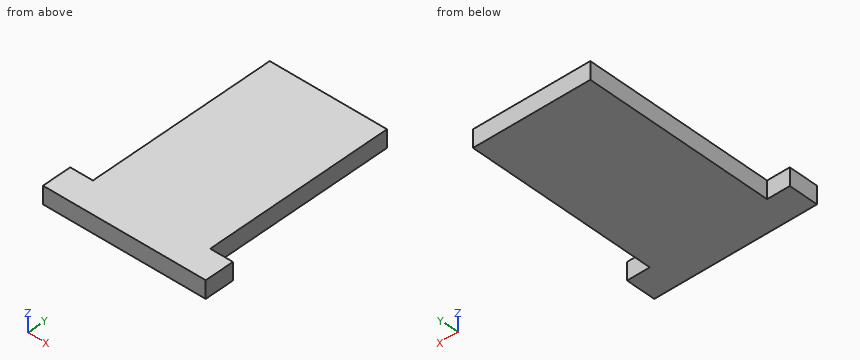
```python
from build123d import *

# Parameters (mm, degrees)
SKETCH1_W           = 8
SKETCH1_H           = 13
BOSS_EXTRUDE1_DEPTH = 0.6
SKETCH2_W           = 11.1
SKETCH2_H           = 2
BOSS_EXTRUDE2_DEPTH = 1.2


with BuildPart() as part:
    # Sketch1 → Boss-Extrude1 (new, symmetric)
    with BuildSketch(Plane.XY):
        Rectangle(SKETCH1_W, SKETCH1_H)
    extrude(amount=BOSS_EXTRUDE1_DEPTH, both=True)

    # Sketch2 → Boss-Extrude2 (add)
    with BuildSketch(Plane.XY.offset(0.6)):
        with Locations((0, -7.5)):
            Rectangle(SKETCH2_W, SKETCH2_H)
    extrude(amount=-BOSS_EXTRUDE2_DEPTH)


solid = part.part
```
The listing builds one solid part. Answer for the finished solid, in the listing's coordinates (mm). Give positions to 0.01 mm unless a question says otherwise; leave off trailing zeros. Loops run counter-clockwise (first coordinate to the right, second up) from the corner with the lowest first, then second, coordinate; pieces in that order, holes last. Notation, with made-up numbers: (-1.75, 84.5) - (17.25, 84.5) arc R15 ccw to (17.25, 102.5) - close; hole circle Ø1 at (2.25, -37). An arc over 180 degrees is marked (long way). Answer as CSV lines item,"result". Start each with the question number.
Item 1: A cutting plane is placed at A-A on z = 0.35. Determine the outline of the cut face in (x, y), then the cut area to 3 significant figures.
Item 2: Each of these flat-tipped pins is pushed along its axis until it touches: pin 1 (0.6 mm diameter, centred on y = -3, z = 0, fed in from +X); pin 2 (0.6 mm diameter, centred on x = 5, z = 0, fed in from +Y); pin 3 (2 mm diameter, centred on x = -4.5, y = -0.5, fed in from +Z). Where does it stop, or does it pass through?
Item 3: Find the intervals of material crossed by line 1 (X direction, y = -1.75, z = -0.15); line 2 (Y direction, x = 5, z = 0), in increasing order. Write a range as from..to.
Item 4: A cutting plane is placed at C-C on y = -2. Determine the outline of the cut face in (x, z), then the cut area to 3 significant figures.
Item 5: A cutting plane is placed at B-B on x = 4.5. Determine the outline of the cut face in (y, z), then the cut area to 3 significant figures.
Found:
1,outline,"(-5.55, -8.5) - (5.55, -8.5) - (5.55, -6.5) - (4, -6.5) - (4, 6.5) - (-4, 6.5) - (-4, -6.5) - (-5.55, -6.5) - close"
1,area,"126 mm^2"
2,pin 1,"stops at x = 4"
2,pin 2,"stops at y = -6.5"
2,pin 3,"stops at z = 0.6"
3,line 1,"x = -4..4"
3,line 2,"y = -8.5..-6.5"
4,outline,"(-4, -0.6) - (4, -0.6) - (4, 0.6) - (-4, 0.6) - close"
4,area,"9.60 mm^2"
5,outline,"(-8.5, -0.6) - (-6.5, -0.6) - (-6.5, 0.6) - (-8.5, 0.6) - close"
5,area,"2.40 mm^2"
